from build123d import *

# Parameters (mm, degrees)
SKETCH1_W                     = 278.2
SKETCH1_H                     = 193.2
SHELL_BLOCK_DEPTH             = 27
SKETCH2_W                     = 273.2
SKETCH2_H                     = 185.8
FRONT_OPENING_DEPTH           = 1.5
SKETCH3_W                     = 273.2
SKETCH3_H                     = 188.2
DISPLAY_POCKET_DEPTH          = 22.5
SKETCH4_W                     = 3
SKETCH4_H                     = 56
VENT_SLOTS_DEPTH              = 4
SKETCH5_W                     = 58
SKETCH5_H                     = 16
CABLE_EXIT_X_SHORT_SIDE_DEPTH = 140.1
SKETCH6_R                     = 1.7
BOLT_HOLES_DEPTH              = 4
KEEP_ONE_HALF_X_DEPTH         = 172.491603293
KEEP_ONE_HALF_X_DEPTH_BACK    = 172.491603293
SKETCH7_W                     = 200
SKETCH7_H                     = 400
KEEP_ONE_QUARTER_Z_DEPTH      = 172.491603293
KEEP_ONE_QUARTER_Z_DEPTH_BACK = 172.491603293
SKETCH8_W                     = 400
SKETCH8_H                     = 200


with BuildPart() as part:
    # Sketch1 → Shell Block (new body)
    with BuildSketch(Plane(origin=(0, 0, 0), x_dir=(1, 0, 0), z_dir=(0, 1, 0))):
        Rectangle(SKETCH1_W, SKETCH1_H)
    extrude(amount=SHELL_BLOCK_DEPTH)

    # Sketch2 → Front Opening (cut)
    with BuildSketch(Plane(origin=(0, 27, 0), x_dir=(1, 0, 0), z_dir=(0, 1, 0))):
        Rectangle(SKETCH2_W, SKETCH2_H)
    extrude(amount=-FRONT_OPENING_DEPTH, mode=Mode.SUBTRACT)

    # Sketch3 → Display Pocket (cut)
    with BuildSketch(Plane(origin=(0, 25.5, 0), x_dir=(1, 0, 0), z_dir=(0, 1, 0))):
        Rectangle(SKETCH3_W, SKETCH3_H)
    extrude(amount=-DISPLAY_POCKET_DEPTH, mode=Mode.SUBTRACT)

    # Sketch4 → Vent Slots (cut)
    with BuildSketch(Plane(origin=(0, 3, 0), x_dir=(1, 0, 0), z_dir=(0, 1, 0))):
        with Locations((-67.5, 56)):
            Rectangle(SKETCH4_W, SKETCH4_H)
        with Locations((-67.5, -56)):
            Rectangle(SKETCH4_W, SKETCH4_H)
        with Locations((-75.5, 56)):
            Rectangle(SKETCH4_W, SKETCH4_H)
        with Locations((-75.5, -56)):
            Rectangle(SKETCH4_W, SKETCH4_H)
        with Locations((-83.5, 56)):
            Rectangle(SKETCH4_W, SKETCH4_H)
        with Locations((-83.5, -56)):
            Rectangle(SKETCH4_W, SKETCH4_H)
        with Locations((-91.5, 56)):
            Rectangle(SKETCH4_W, SKETCH4_H)
        with Locations((-91.5, -56)):
            Rectangle(SKETCH4_W, SKETCH4_H)
        with Locations((-99.5, 56)):
            Rectangle(SKETCH4_W, SKETCH4_H)
        with Locations((-99.5, -56)):
            Rectangle(SKETCH4_W, SKETCH4_H)
        with Locations((-107.5, 56)):
            Rectangle(SKETCH4_W, SKETCH4_H)
        with Locations((-107.5, -56)):
            Rectangle(SKETCH4_W, SKETCH4_H)
        with Locations((-115.5, 56)):
            Rectangle(SKETCH4_W, SKETCH4_H)
        with Locations((-115.5, -56)):
            Rectangle(SKETCH4_W, SKETCH4_H)
        with Locations((-123.5, 56)):
            Rectangle(SKETCH4_W, SKETCH4_H)
        with Locations((-123.5, -56)):
            Rectangle(SKETCH4_W, SKETCH4_H)
    extrude(amount=-VENT_SLOTS_DEPTH, mode=Mode.SUBTRACT)

    # Sketch5 → Cable Exit (-X short side) (cut)
    with BuildSketch(Plane(origin=(0, 0, 0), x_dir=(0, 0, -1), z_dir=(1, 0, 0))):
        with Locations((0, 13)):
            Rectangle(SKETCH5_W, SKETCH5_H)
    extrude(amount=-CABLE_EXIT_X_SHORT_SIDE_DEPTH, mode=Mode.SUBTRACT)

    # Sketch6 → Bolt Holes (cut)
    with BuildSketch(Plane(origin=(0, 3, 0), x_dir=(1, 0, 0), z_dir=(0, 1, 0))):
        with Locations(Location((-40, 18, 0), (0, 0, 270))):
            Circle(SKETCH6_R)
        with Locations(Location((-40, 88, 0), (0, 0, 270))):
            Circle(SKETCH6_R)
        with Locations(Location((40, 18, 0), (0, 0, 270))):
            Circle(SKETCH6_R)
        with Locations(Location((40, 88, 0), (0, 0, 270))):
            Circle(SKETCH6_R)
        with Locations(Location((-52, 40, 0), (0, 0, 270))):
            Circle(SKETCH6_R)
        with Locations(Location((-52, 66, 0), (0, 0, 270))):
            Circle(SKETCH6_R)
        with Locations(Location((52, 40, 0), (0, 0, 270))):
            Circle(SKETCH6_R)
        with Locations(Location((52, 66, 0), (0, 0, 270))):
            Circle(SKETCH6_R)
        with Locations(Location((-12, -82, 0), (0, 0, 270))):
            Circle(SKETCH6_R)
        with Locations(Location((12, -82, 0), (0, 0, 270))):
            Circle(SKETCH6_R)
        with Locations(Location((124, -12, 0), (0, 0, 270))):
            Circle(SKETCH6_R)
        with Locations(Location((124, 12, 0), (0, 0, 270))):
            Circle(SKETCH6_R)
        with Locations(Location((-12, -12, 0), (0, 0, 270))):
            Circle(SKETCH6_R)
        with Locations(Location((-12, 12, 0), (0, 0, 270))):
            Circle(SKETCH6_R)
        with Locations(Location((12, -12, 0), (0, 0, 270))):
            Circle(SKETCH6_R)
        with Locations(Location((12, 12, 0), (0, 0, 270))):
            Circle(SKETCH6_R)
        with Locations(Location((-110, 12, 0), (0, 0, 270))):
            Circle(SKETCH6_R)
        with Locations(Location((-110, -12, 0), (0, 0, 270))):
            Circle(SKETCH6_R)
        with Locations(Location((-86, 12, 0), (0, 0, 270))):
            Circle(SKETCH6_R)
        with Locations(Location((-86, -12, 0), (0, 0, 270))):
            Circle(SKETCH6_R)
    extrude(amount=-BOLT_HOLES_DEPTH, mode=Mode.SUBTRACT)

    # Sketch7 → Keep one half (X) (cut, two sides: drawn at the far end of the back side and taken through both)
    with BuildSketch(Plane(origin=(0, 0, 0), x_dir=(1, 0, 0), z_dir=(0, 1, 0)).offset(-KEEP_ONE_HALF_X_DEPTH_BACK)):
        with Locations((100, 0)):
            Rectangle(SKETCH7_W, SKETCH7_H)
    extrude(amount=KEEP_ONE_HALF_X_DEPTH + KEEP_ONE_HALF_X_DEPTH_BACK, mode=Mode.SUBTRACT)

    # Sketch8 → Keep one quarter (Z) (cut, two sides: drawn at the far end of the back side and taken through both)
    with BuildSketch(Plane(origin=(0, 0, 0), x_dir=(1, 0, 0), z_dir=(0, 1, 0)).offset(-KEEP_ONE_QUARTER_Z_DEPTH_BACK)):
        with Locations((0, 100)):
            Rectangle(SKETCH8_W, SKETCH8_H)
    extrude(amount=KEEP_ONE_QUARTER_Z_DEPTH + KEEP_ONE_QUARTER_Z_DEPTH_BACK, mode=Mode.SUBTRACT)


solid = part.part
Design review of the part built by this model. Coordinates are the model's own, in mm. Give positions to 0.01 mm unless a question says otherwise; leave off trailing zeros. Loops run counter-clockwise (first coordinate to the right, second up) from the corner with the lowest first, then second, coordinate; pieces in that order, holes last. Notation, with made-up numbers: M -13,82 L 11,82 A11 ccw 11,96 Z; hole C 58,33 d11. An arc over 180 degrees is marked long. Answer as a JSON object with one key per item and string values.
Item 1: Mouldability with a two-part tool opening along X and no side actions: class faces 1 (the face through (-12.65, 1.52, 13.57)), 2 (the face through (-139.1, 13, 60)) as pulls with the +X half, pulls with the -X half, needs draft (parallel to the pull), parting line crosses it, or undercut.
Output values:
{"face 1": "undercut", "face 2": "pulls with the -X half"}
Item 2: We need section B-B (z = 12). State the section outline as (x, y) points, and give its area (3 significant figures).
Output values:
{"outline": "M -139.1,0 L -111.7,0 L -111.7,3 L -136.6,3 L -136.6,5 L -139.1,5 Z; M -139.1,21 L -136.6,21 L -136.6,27 L -139.1,27 Z; M -108.3,0 L -87.7,0 L -87.7,3 L -108.3,3 Z; M -84.3,0 L -13.7,0 L -13.7,3 L -84.3,3 Z; M -10.3,0 L 0,0 L 0,3 L -10.3,3 Z", "area": "407 mm2"}
Item 3: We need section D-D (y = 22.75). State the section outline as (x, z) points.
Output values:
{"outline": "M -139.1,0 L -136.6,0 L -136.6,94.1 L 0,94.1 L 0,96.6 L -139.1,96.6 Z"}
Item 4: We need section A-A (x = -12). State the section outline as (y, z) points, and give its area (3 significant figures).
Output values:
{"outline": "M 0,0 L 3,0 L 3,10.3 L 0,10.3 Z; M 0,13.7 L 3,13.7 L 3,80.3 L 0,80.3 Z; M 0,83.7 L 3,83.7 L 3,94.1 L 25.5,94.1 L 25.5,92.9 L 27,92.9 L 27,96.6 L 0,96.6 Z", "area": "331 mm2"}
Item 5: We need section C-C (z = 24). State the section outline as (x, y) points.
Output values:
{"outline": "M -139.1,0 L 0,0 L 0,3 L -136.6,3 L -136.6,5 L -139.1,5 Z; M -139.1,21 L -136.6,21 L -136.6,27 L -139.1,27 Z"}
Item 6: Wall thickness on line 1 along X through (y, z) = (2.2, 12); line 2 along Z through (x, y) = (-110, 1.6); line 3 along X through (y, z) = (4.25, 70): over which ranges is each line inside the solid? List them lowest first.
Output values:
{"line 1": "x = -139.1 to -111.7, -108.3 to -87.7, -84.3 to -13.7, -10.3 to 0", "line 2": "z = 0 to 10.3, 13.7 to 96.6", "line 3": "x = -139.1 to -136.6"}
Item 7: For P1, Ø12, axis at y = 11, z = 54, coming from the +X side; P2, Ø10, axis at x = -118.5, z = 77.5, coming from the +Y side; P3, Ø3, axis at x = -31, y = 14.5, coming from the -Z side, all flat-tipped, find the tip position at first contact; note any pin that passes through.
Output values:
{"P1": "stops at x = -136.6", "P2": "stops at y = 3", "P3": "stops at z = 94.1"}
